For this review, take the finished solid that the model builds, in its own axes (mm). A direction names the side the tool comes from. Give positions to 0.01 mm unless a question says otherwise; leave off trailing zeros. Order: outer loops, then holes, each group sorted by start corner. A loop starts at its lowest first (then second) coordinate and runs counter-clockwise, first axis right, second up. Notation, with made-up numbers: M 4.5,-39.5 L 31.5,-39.5 A20 ccw 31.5,-27.5 Z; hole C 26,21.5 d6. An arc over 180 degrees is marked long. Use CSV: the item, a comma, the result in double quotes. Start each with the question number.
(1) Wall thickness on L1, parallel to Y at x = -6.9, z = 0; L2, parallel to X at y = 12, z = -2.5; L3, parallel to Z at x = -4.5, y = 10.5: over which ranges is each line inside the solid? List them lowest first. Write a range as from..to.
(2) Draft analysis for pull direction Y (two halves, no side actions). For faces 1 (the face through (-0.465, -5.072, 2.965)), 2 (the face through (-7.874, 18.761, 2.463)), 3 (the face through (2, 6, -2)), state which applies: pulls with the +Y half, pulls with the -Y half, needs draft (parallel to the pull), parting line crosses it, or undercut.
(3) Tool access review of faces 4 (the face through (-8.5, -17, 3)), 5 (the face through (-0.465, 5.072, -2.965)), 6 (the face through (0.986, -7.808, 1.025)), 7 (the face through (-3, 0, -7)): name each direction out of +Z, -Z, +X, -X, +Y, -Y from which nothing blocks a thin tool from reaching the whole face with its end or side.
(4) Consider section B-B (z = 0). Write out the cut boundary in (x, y) (3 decimals).
(5) Clearance check with flat-ended pins moving along their axes: P1, Ø8, axis at y = -9.5, z = -8, coming from the +X side; P2, Ø4, axis at x = -5.5, z = 0.5, coming from the +Y side; P3, Ø2, axis at x = -2.5, y = 12.5, coming from the +Z side. State where each tip first meets the part, or that it passes through.
(6) Consider section C-C (y = 0). Write out the cut boundary in (x, z) (3 decimals).
(7) Consider section A-A (x = 0.5). Write out the cut boundary in (y, z) (3 decimals), and give its area (3 significant figures).
(8) Consider section D-D (x = -2.25). Write out the cut boundary in (y, z) (3 decimals), and give its area (3 significant figures).
Autodesk Inventor part; units mm, degrees
ref_plane "YZ Plane" through (0, 0, 0) normal (1, 0, 0) x (0, 1, 0)
ref_plane "XZ Plane" through (0, 0, 0) normal (0, 1, 0) x (-1, 0, 0)
ref_plane "XY Plane" through (0, 0, 0) normal (0, 0, 1) x (1, 0, 0)
sketch "Sketch1" plane through (0, 0, 0) normal (0, 1, 0) x (-1, 0, 0)
  line L0 (0, 0) -> (3, 0) construction
  line L1 (3, 0) -> (3, -5.875) construction
  line L2 (3, -5.875) -> (0, -5.875) construction
  line L3 (0, -5.875) -> (0, 0) construction
  line L4 (0, -5.875) -> (3, -5.875)
  line L5 (3, -5.875) -> (3, -23)
  line L6 (3, -23) -> (0, -23)
  line L7 (0, -23) -> (0, -5.875)
  line L8 (8.5, -23) -> (-1.5, -23) construction
  line L9 (-1.5, -23) -> (-1.5, -17)
  line L10 (-1.5, -17) -> (8.5, -17)
  line L11 (8.5, -17) -> (8.5, -23)
  line L12 (-1.5, -21) -> (8.5, -18.7831)
  line L13 (-1.5, -19.4636) -> (8.5, -17.2466)
  line L14 (3, -5.875) -> (5, -5.875)
  line L15 (5, -5.875) -> (5, -9.875)
  line L16 (5, -9.875) -> (3, -9.875)
  line L17 (3, -9.875) -> (3, -5.875)
  line L18 (0, -5.875) -> (-2, -5.875)
  line L19 (-2, -5.875) -> (-2, -7.875)
  line L20 (-2, -7.875) -> (0, -7.875)
  line L21 (0, -7.875) -> (0, -5.875)
  point P0 (3, -17)
  point P1 (0, -17)
  point P2 (0, -19.131)
  point P3 (3, -18.466)
  point P4 (3, -9.875)
  point P5 (0, -7.875)
  dimension "d21" = 3
  dimension "d22" = 5.875
  dimension "d24" = 1.5
  dimension "d25" = 10
  dimension "d26" = 6
  dimension "d27" = 2
  dimension "d29" = 21
  dimension "d30" = 1.5
  dimension "d34" = 2
  dimension "d35" = 4
  dimension "d36" = 2
  dimension "d37" = 2
  dimension "d38" = 12.5
revolve "Revolution1" add sketch "Sketch1" angle 360 about axis through (0, 0, 0) along (-1, 0, 0) contours L4 L5 L10 L7 | L7 L20 L19 L18 | L10 L5 L13 L7 | L10 L11 L13 L5 | L13 L5 L12 L7 | L7 L12 L9 L13 | L13 L11 L12 L5
sketch "Sketch5" plane through (-3, 0, 0) normal (-1, 0, 0) x (0, 0, 1)
  line L0 (0, 0) -> (-5.875, 0) construction
  line L1 (-5.875, 3.3919) -> (0, 6.7839)
  line L2 (0, 6.7839) -> (5.875, 3.3919)
  line L3 (5.875, 3.3919) -> (5.875, -3.3919)
  line L4 (5.875, -3.3919) -> (0, -6.7839)
  line L5 (0, -6.7839) -> (-5.875, -3.3919)
  line L6 (-5.875, -3.3919) -> (-5.875, 3.3919)
  circle A0 centre (0, 0) radius 5.875
  circle A1 centre (0, 0) radius 17
  circle A2 centre (0, 0) radius 5.875
extrude "Extrusion4" cut sketch "Sketch5" along normal through all both and the other way through all contours L1 A0 L6 | L1 L2 A0 | A0 | A0 L5 L6 | L2 L3 A0 | A0 L4 L5 | L3 L4 A0
fillet "Fillet4" radius 2 6 edges at (-0.5, -3.3919, -5.875) (-0.5, 3.3919, -5.875) (-0.5, 6.7839, 0) (-0.5, -6.7839, 0) (-0.5, -3.3919, 5.875) (-0.5, 3.3919, 5.875)
properties part number "Clutch" material "Stainless Steel"
Check result:
1,L1,"y = -19.14..-17, 17..19.14"
1,L2,"x = -3..0"
1,L3,"z = -16.63..-13.37, 13.37..16.63"
2,face 1,"undercut"
2,face 2,"parting line crosses it"
2,face 3,"needs draft"
3,face 4,"+Z, -Z, -X, +Y, -Y"
3,face 5,"+X, -X"
3,face 6,"+X"
3,face 7,"-X"
4,outline,"M -8.5,-18.783 L 1.5,-21 L 1.5,-19.464 L 0,-19.131 L 0,-7.875 L 2,-7.875 L 2,-6.474 L -3,-6.474 L -3,-17 L -8.5,-17 Z; M -8.5,17 L -3,17 L -3,6.474 L 2,6.474 L 2,7.875 L 0,7.875 L 0,19.131 L 1.5,19.464 L 1.5,21 L -8.5,18.783 Z"
5,P1,"stops at x = 0"
5,P2,"stops at y = 19.89"
5,P3,"stops at z = 16.55"
6,outline,"M -8.5,-18.783 L 1.5,-21 L 1.5,-19.464 L 0,-19.131 L 0,-7.875 L 2,-7.875 L 2,-5.875 L -3,-5.875 L -3,-17 L -8.5,-17 Z; M -8.5,17 L -3,17 L -3,5.875 L 2,5.875 L 2,7.875 L 0,7.875 L 0,19.131 L 1.5,19.464 L 1.5,21 L -8.5,18.783 Z"
7,outline,"C 0,0 d41.557; C 0,0 d15.75; hole C 0,0 d38.484; hole M -6.207,-1 L -3.969,-4.875 A2 ccw -2.237,-5.875 L 2.237,-5.875 A2 ccw 3.969,-4.875 L 6.207,-1 A2 ccw 6.207,1 L 3.969,4.875 A2 ccw 2.237,5.875 L -2.237,5.875 A2 ccw -3.969,4.875 L -6.207,1 A2 ccw Z"
7,area,"270 mm^2"
8,outline,"C 0,0 d40.337; hole M -6.207,-1 L -3.969,-4.875 A2 ccw -2.237,-5.875 L 2.237,-5.875 A2 ccw 3.969,-4.875 L 6.207,-1 A2 ccw 6.207,1 L 3.969,4.875 A2 ccw 2.237,5.875 L -2.237,5.875 A2 ccw -3.969,4.875 L -6.207,1 A2 ccw Z"
8,area,"1,160 mm^2"
